Verification items for the finished model (mm, model axes). Round coordinates to 2 decimals unless told otherwise and drop trailing zeros. Loops run counter-clockwise (first coordinate to the right, second up) from the corner with the lowest first, then second, coordinate; pieces in that order, holes last.
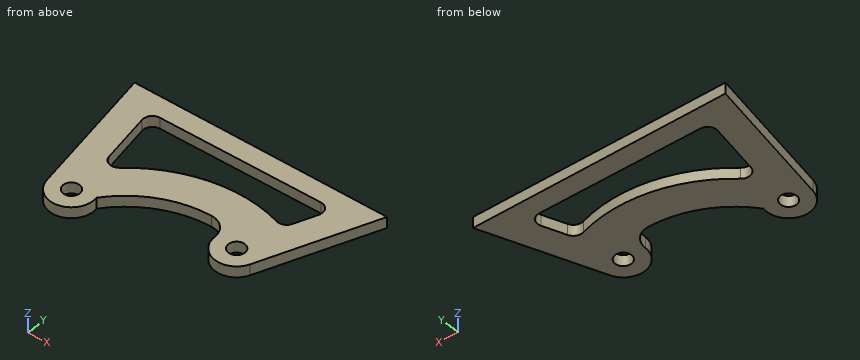
from build123d import *

# Parameters (mm, degrees)
SKETCH1_R           = 4.5
BOSS_EXTRUDE1_DEPTH = 6


with BuildPart() as part:
    # Sketch1 → Boss-Extrude1 (new body)
    with BuildSketch(Plane.XY):
        with BuildLine():
            Line((538.087061333, -362.632518419), (399.195756936, -361.813220805))
            Line((399.195756936, -361.813220805), (411.770395569, -435.296905236))
            ThreePointArc((411.770395569, -435.296905236), (425.804925586, -445.068271221), (435.358389017, -430.884514226))
            ThreePointArc((435.358389017, -430.884514226), (455.39069986, -414.804899258), (480.456241604, -409.186526513))
            ThreePointArc((480.456241604, -409.186526513), (487.46072005, -412.122937916), (490.381767865, -419.133837281))
            ThreePointArc((490.381767865, -419.133837281), (500.126063062, -430.857058146), (513.510317286, -423.560008386))
            Line((513.510317286, -423.560008386), (538.087061333, -362.632518419))
        make_face()
        with Locations((423.598466956, -433.272867865)):
            Circle(SKETCH1_R, mode=Mode.SUBTRACT)
        with Locations((502.381603037, -419.070941762)):
            Circle(SKETCH1_R, mode=Mode.SUBTRACT)
        with BuildLine():
            ThreePointArc((510.342575031, -372.949836208), (514.486982235, -375.152714664), (514.979539302, -379.820280635))
            Line((514.979539302, -379.820280635), (510.209986836, -391.644339161))
            ThreePointArc((510.209986836, -391.644339161), (507.666881017, -394.314352508), (503.985021193, -394.515018193))
            ThreePointArc((503.985021193, -394.515018193), (465.150215538, -392.093753549), (430.277606866, -409.353701903))
            ThreePointArc((430.277606866, -409.353701903), (425.309411141, -410.309514397), (422.050350523, -406.439750816))
            Line((422.050350523, -406.439750816), (417.319428607, -378.793185112))
            ThreePointArc((417.319428607, -378.793185112), (418.425701646, -374.726231434), (422.247791685, -372.949836208))
            Line((422.247791685, -372.949836208), (510.342575031, -372.949836208))
        make_face(mode=Mode.SUBTRACT)
    extrude(amount=-BOSS_EXTRUDE1_DEPTH)


solid = part.part
1. Section check B-B (y = -422). Enter the section's corners in (x, z) (3 decimals).
2. Section check A-A (x = 453). Enter the section's corners in (y, z), then the cut area to 3 significant figures.
3. Section check C-C (z = -4.05). Enter the section's corners in (x, y).
4. Section check D-D (y = -401). Enter the section's corners in (x, z), then the cut area to 3 significant figures.
5. Gauge pin test, flat ends, axial feed: P1, Ø1, axis at x = 498.5, z = -3, coming from the +Y side; P2, Ø2, axis at x = 496.5, z = -1, coming from the -Y side; P3, Ø1.5, axis at x = 447, z = -3.5, coming from the +Y side. Record the tip position at first contact, or that the pin passes through.
6. Scan lines: L1, parallel to X at y = -418, z = -2.65; L2, parallel to X at y = -421.5, z = -2.7; L3, parallel to X at y = -374, z = -3.1. Record each from-to range of solid material in increasing order.
Taken from the geometry:
1. outline: (409.495, -6) - (444.082, -6) - (444.082, 0) - (409.495, 0) - close; (490.745, -6) - (498.965, -6) - (498.965, 0) - (490.745, 0) - close; (505.798, -6) - (514.14, -6) - (514.14, 0) - (505.798, 0) - close
2. outline: (-416.03, -6) - (-395.62, -6) - (-395.62, 0) - (-416.03, 0) - close; (-372.95, -6) - (-362.13, -6) - (-362.13, 0) - (-372.95, 0) - close
2. area: 187 mm2
3. outline: (399.2, -361.81) - (411.77, -435.3) arc R12 ccw (long way) to (435.36, -430.88) arc R56.84 cw to (480.46, -409.19) arc R10 cw to (490.38, -419.13) arc R12 ccw to (513.51, -423.56) - (538.09, -362.63) - close; hole (417.32, -378.79) - (422.05, -406.44) arc R5 ccw to (430.28, -409.35) arc R75.41 cw to (503.99, -394.52) arc R5 ccw to (510.21, -391.64) - (514.98, -379.82) arc R5 ccw to (510.34, -372.95) - (422.25, -372.95) arc R5 ccw to start; hole circle Ø9 at (423.6, -433.27); hole circle Ø9 at (502.38, -419.07)
4. outline: (405.9, -6) - (421.12, -6) - (421.12, 0) - (405.9, 0) - close; (441.84, -6) - (522.61, -6) - (522.61, 0) - (441.84, 0) - close
4. area: 576 mm2
5. P1: stops at y = -362.4
5. P2: stops at y = -430.03
5. P3: stops at y = -362.09
6. L1: x = 408.81 to 449.63, 490.31 to 498.01, 506.75 to 515.75
6. L2: x = 409.41 to 444.7, 490.63 to 498.59, 506.17 to 514.34
6. L3: x = 401.28 to 419.18, 513.41 to 533.5
